```python
from build123d import *

# Parameters (mm, degrees)
F1_DEPTH  = 13.5
F3_R      = 12.6
F4_DEPTH  = 6.5
F6_DEPTH  = 15
F7_DEPTH  = 6.5
F8_DEPTH  = 70
F10_DEPTH = 90
F12_DEPTH = 15
F17_R     = 3.25
F18_DEPTH = 93.701
F20_R     = 7
F21_DEPTH = 90
F22_R     = 7
F23_DEPTH = 0.16
F24_R     = 7
F25_DEPTH = 0.16
F26_R     = 1.3
F27_DEPTH = 12.5


with BuildPart() as f1:
    # F0 (on Top) → F1 (new body)
    with BuildSketch(Plane.XY):
        with BuildLine():
            ThreePointArc((-1, -9.9498743711), (-10, 0), (-1, 9.9498743711))
            Line((-1, 9.9498743711), (-1, 12.5602547745))
            ThreePointArc((-1, 12.5602547745), (-12.6, 0), (-1, -12.5602547745))
            Line((-1, -12.5602547745), (-1, -9.9498743711))
        make_face()
        with BuildLine():
            ThreePointArc((-1, -9.9498743711), (6.7082039325, -7.4161984871), (10, 0))
            ThreePointArc((10, 0), (6.7082039325, 7.4161984871), (-1, 9.9498743711))
            ThreePointArc((-1, 9.9498743711), (-10, 0), (-1, -9.9498743711))
        make_face()
    extrude(amount=-F1_DEPTH)

    # F3 (on offset) → F4 (join)
    with BuildSketch(Plane.XY.offset(-20)):
        Circle(F3_R)
    extrude(amount=F4_DEPTH)

    # F5 (on Front) → F6 (cut, symmetric)
    with BuildSketch(Plane.XZ):
        Polygon((12.6, -13.5), (-1, -13.5), (12.6, -20), align=None)
    extrude(amount=F6_DEPTH, both=True, mode=Mode.SUBTRACT)

    # F7 (add): a face of the model
    f7_faces = [f1.faces().sort_by_distance(p)[0] for p in [
        (3.7091534646, 0, -13.5),
    ]]
    extrude(f7_faces, amount=F7_DEPTH)

    # F8 (add): a face of the model
    f8_faces = [f1.faces().sort_by_distance(p)[0] for p in [
        (0, 0, -20),
    ]]
    extrude(f8_faces, amount=F8_DEPTH)

    # F9 (on face) → F10 (cut)
    with BuildSketch(Plane(origin=(0, 0, -90), x_dir=(1, 0, 0), z_dir=(0, 0, -1))):
        with BuildLine():
            Line((10.4, 7.1133676975), (10.4, 0))
            Line((10.4, 0), (10.4, -7.1133676975))
            ThreePointArc((10.4, -7.1133676975), (12.0374415886, -3.7229020938), (12.6, 0))
            ThreePointArc((12.6, 0), (12.0374415886, 3.7229020938), (10.4, 7.1133676975))
        make_face()
    extrude(amount=-F10_DEPTH, mode=Mode.SUBTRACT)

    # F11 (on face) → F12 (cut)
    with BuildSketch(Plane(origin=(0, 0, -90), x_dir=(1, 0, 0), z_dir=(0, 0, -1))):
        with BuildLine():
            ThreePointArc((8.6, 6.5329931884), (-10.8, 0), (8.6, -6.5329931884))
            Line((8.6, -6.5329931884), (8.6, 6.5329931884))
        make_face()
    extrude(amount=-F12_DEPTH, mode=Mode.SUBTRACT)

    # F13 (on face) → F16 section 0
    with BuildSketch(Plane.XY):
        with BuildLine():
            Line((6, 0), (6, 4.069705149))
            ThreePointArc((6, 4.069705149), (0, 7.25), (-6, 4.069705149))
            Line((-6, 4.069705149), (-6, 0))
            Line((-6, 0), (-6, -4.069705149))
            ThreePointArc((-6, -4.069705149), (0, -7.25), (6, -4.069705149))
            Line((6, -4.069705149), (6, 0))
        make_face()
    # F15 (on offset) → F16 section 1
    with BuildSketch(Plane.XY.offset(3.7)):
        with BuildLine():
            Line((5, 0), (5, 3.75))
            ThreePointArc((5, 3.75), (0, 6.25), (-5, 3.75))
            Line((-5, 3.75), (-5, 0))
            Line((-5, 0), (-5, -3.75))
            ThreePointArc((-5, -3.75), (0, -6.25), (5, -3.75))
            Line((5, -3.75), (5, 0))
        make_face()
    loft()

    # F17 (on offset) → F18 (cut, through all)
    with BuildSketch(Plane.XY.offset(3.7)):
        Circle(F17_R)
    extrude(amount=-F18_DEPTH, mode=Mode.SUBTRACT)

    # F20 (on offset) → F21 (cut)
    with BuildSketch(Plane.XY.offset(-3)):
        Circle(F20_R)
    extrude(amount=-F21_DEPTH, mode=Mode.SUBTRACT)

    # F22 (on face) → F23 (join)
    with BuildSketch(Plane(origin=(0, 0, -75), x_dir=(1, 0, 0), z_dir=(0, 0, -1))):
        Circle(F22_R)
    extrude(amount=-F23_DEPTH)

    # F24 (on offset) → F25 (join)
    with BuildSketch(Plane.XY.offset(-3)):
        Circle(F24_R)
    extrude(amount=F25_DEPTH)

    # F26 (on Front) → F27 (cut, symmetric)
    with BuildSketch(Plane.XZ):
        with Locations((2, -11.5)):
            Circle(F26_R)
    extrude(amount=F27_DEPTH, both=True, mode=Mode.SUBTRACT)


solid = f1.part
```
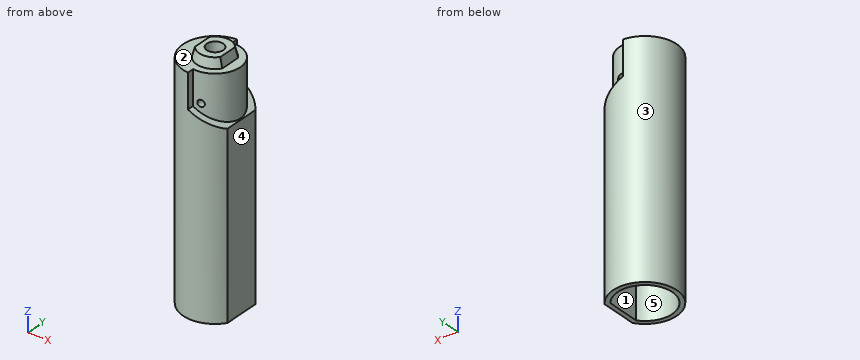
Geometry check sheet. Reference: the model listing, model coordinates, mm. Face numbers are marked on the shaded views. A direction names the side the tool comes from. Coordinates: 2 decimals unless noted, no trailing zeros. Loops run counter-clockwise (first coordinate to the right, second up) from the corner with the lowest first, then second, coordinate; pieces in that order, holes last. Notation, with made-up numbers: (65, -29.5) -> (90, -29.5) arc R22 ccw to (90, -0.5) -> close; hole circle Ø10 at (-29, 46). An arc over 180 degrees is marked (long way). Put each result on its own line as item: value.
1) Thickness scan on line 1 (Y direction, x = -0.25, z = -69.5); line 2 (Z direction, x = 2, y = 1.25); line 3 (Z direction, x = 3.25, y = -0.5). Record the ranges inside material, lowest first.
Result set:
line 1: y = -12.6 to -7, 7 to 12.6
line 2: z = -75 to -74.84, -3 to -2.84
line 3: z = -75 to -74.84, -3 to 3.7
2) Cross-section at C-C on z = -56.5. Record the boundary of the cut face in (x, y), plus the area to 3 significant figures.
Result set:
outline: (10.4, -7.11) -> (10.4, 7.11) arc R12.6 ccw (long way) to start; hole circle Ø14 at (0, 0)
area: 324 mm^2
3) Release check for a two-part mould opening along Y. For the marked faces 3, 4 and 5 record: released by +Y, released by -Y, zero draft, split by the parting line, or undercut.
Result set:
face 3: split by the parting line
face 4: zero draft
face 5: undercut
4) Cross-section at A-A on z = -11.5. Record the boundary of the cut face in (x, y).
Result set:
outline: (-1, -12.56) -> (-1, -9.95) arc R10 ccw to (0.7, -9.98) -> (0.7, -6.96) arc R7 cw (long way) to (0.7, 6.96) -> (0.7, 9.98) arc R10 ccw to (-1, 9.95) -> (-1, 12.56) arc R12.6 ccw to start; (3.3, -9.44) arc R10 ccw to (3.3, 9.44) -> (3.3, 6.17) arc R7 cw to (3.3, -6.17) -> close
5) Cross-section at B-B on z = -76. Record the boundary of the cut face in (x, y).
Result set:
outline: (10.4, -7.11) -> (10.4, 7.11) arc R12.6 ccw (long way) to start; hole (8.6, -6.53) -> (8.6, 6.53) arc R10.8 ccw (long way) to start
6) Gauge pin test, flat ends, axial feed: pin 1 Ø1.5 at (x, z) = (5, -47.5) entering from +Y; pin 2 Ø1.5 at (y, z) = (2.5, -15.5) entering from -X; pin 3 Ø6 at (x, z) = (-6.5, -75.5) entering from +Y. Record the tip position at first contact, or that the pin passes through.
Result set:
pin 1: stops at y = 11.86
pin 2: stops at x = -12.48
pin 3: stops at y = 12.1
7) Tool access check on the marked faces 1 and 2. Record the directions out of +Z, -Z, +X, -X, +Y, -Y that give a thin tool (end or side, any length) a straight path to the whole face; none if there is none.
Result set:
face 1: -Z
face 2: +Z
